from build123d import *

# Parameters (mm, degrees)
SKETCH1_W           = 97.5
SKETCH1_H           = 12
BOSS_EXTRUDE1_DEPTH = 3
SKETCH2_W           = 103.5
SKETCH2_H           = 18
SKETCH2_W_2         = 97.5
SKETCH2_H_2         = 12
BOSS_EXTRUDE2_DEPTH = 9


with BuildPart() as part:
    # Sketch1 → Boss-Extrude1 (new body)
    with BuildSketch(Plane.XY):
        with Locations((48.75, 6)):
            Rectangle(SKETCH1_W, SKETCH1_H)
    extrude(amount=BOSS_EXTRUDE1_DEPTH)

    # Sketch2 → Boss-Extrude2 (add)
    with BuildSketch(Plane(origin=(0, 0, 0), x_dir=(-1, 0, 0), z_dir=(0, 0, -1))):
        with Locations((-48.75, 6)):
            Rectangle(SKETCH2_W, SKETCH2_H)
        with Locations((-48.75, 6)):
            Rectangle(SKETCH2_W_2, SKETCH2_H_2, mode=Mode.SUBTRACT)
    extrude(amount=-BOSS_EXTRUDE2_DEPTH)


solid = part.part
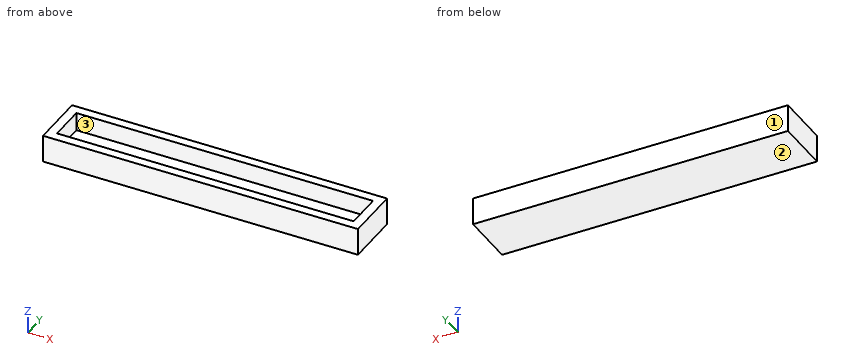
Verification items for the finished model (mm, model axes). Face numbers are marked on the shaded views. Coordinates: 2 decimals unless noted, no trailing zeros. Order: outer loops, then holes, each group sorted by start corner. A loop starts at its lowest first (then second) coordinate and runs counter-clockwise, first axis right, second up.
1. Sectioned sample at C-C, the plane x = 56.5. Record the cut outline in (y, z), and give its area (3 significant figures).
Results found:
outline: (-3, 0) - (15, 0) - (15, 9) - (12, 9) - (12, 3) - (0, 3) - (0, 9) - (-3, 9) - close
area: 90.0 mm2
2. Sectioned sample at B-B, the plane z = 5.5. Record the cut outline in (x, y).
Results found:
outline: (-3, -3) - (100.5, -3) - (100.5, 15) - (-3, 15) - close; hole (0, 0) - (97.5, 0) - (97.5, 12) - (0, 12) - close
3. Sectioned sample at A-A, the plane y = 7. Record the cut outline in (x, z), and give its area (4 significant figures).
Results found:
outline: (-3, 0) - (100.5, 0) - (100.5, 9) - (97.5, 9) - (97.5, 3) - (0, 3) - (0, 9) - (-3, 9) - close
area: 346.5 mm2
4. Scan lines: line 1 (X direction, y = 2.25, z = 7); line 2 (Y direction, x = 30.5, z = 3.75); line 3 (Z direction, x = 64.5, y = 1). Record each from-to range of solid material in increasing order.
Results found:
line 1: x = -3 to 0, 97.5 to 100.5
line 2: y = -3 to 0, 12 to 15
line 3: z = 0 to 3
5. Release check for a two-part mould opening along Y. For the marked faces 1, 2 and 3 record: +Y half, -Y half, draft (parallel to the pull), parting line (faces both ways), or undercut.
Results found:
face 1: +Y half
face 2: draft
face 3: undercut
